The figure shows three views and two pictorial views of one solid part (mm, origin at its lowest corner). Answer the questions. A direction names the side the tool comes from. Round coordinates to 2 decimals unless told otherwise and drop trailing zeros. Order: outer loops, then holes, each group sorted by start corner. A loop starts at its lowest first (then second) coordinate and runs counter-clockwise, first axis right, second up. Notation, with made-up numbers: M 27.5,-12.75 L 53.5,-12.75 A24 cw 53.5,13.25 Z; hole C 38.25,0.5 d8. An arc over 180 degrees is marked long. Answer as CSV lines item,"result".
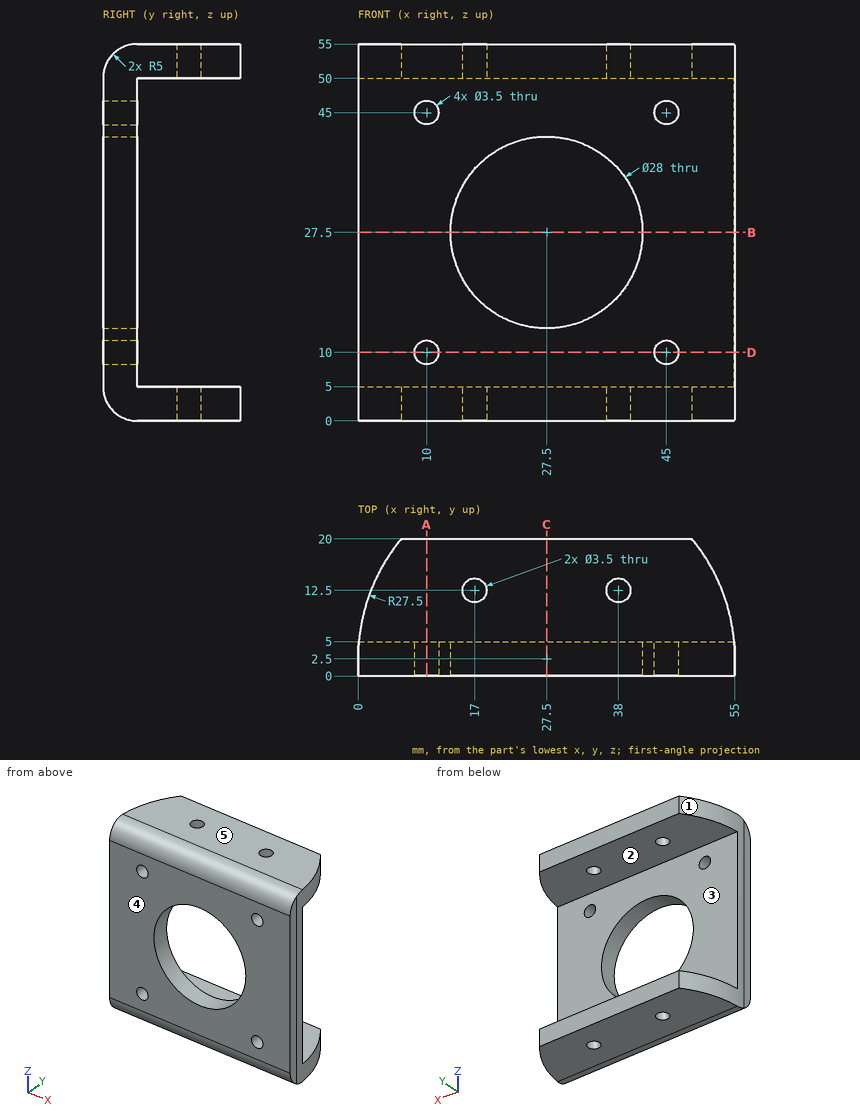
Item 1: A cutting plane is placed at D-D, the plane z = 10. Determine the outline of the cut face in (x, y), and give its area (3 significant figures).
Ans:
outline,"M 0,0 L 8.25,0 L 8.25,5 L 0.11,5 A27.5 ccw 0,2.5 Z; M 11.75,0 L 43.25,0 L 43.25,5 L 11.75,5 Z; M 46.75,0 L 55,0 L 55,2.5 A27.5 ccw 54.89,5 L 46.75,5 Z"
area,"240 mm2"
Item 2: A cutting plane is placed at A-A, the plane x = 10. Determine the outline of the cut face in (y, z), and give its area (3 significant figures).
Ans:
outline,"M 0,5 A5 ccw 5,0 L 20,0 L 20,5 L 5,5 L 5,8.25 L 0,8.25 Z; M 0,11.75 L 5,11.75 L 5,43.25 L 0,43.25 Z; M 0,46.75 L 5,46.75 L 5,50 L 20,50 L 20,55 L 5,55 A5 ccw 0,50 Z"
area,"379 mm2"
Item 3: A cutting plane is placed at C-C, the plane x = 27.5. Determine the outline of the cut face in (y, z).
Ans:
outline,"M 0,5 A5 ccw 5,0 L 20,0 L 20,5 L 5,5 L 5,13.5 L 0,13.5 Z; M 0,41.5 L 5,41.5 L 5,50 L 20,50 L 20,55 L 5,55 A5 ccw 0,50 Z"
Item 4: Flat-ended cylindrical pins translate along their axes: pin 1 (22.5 mm diameter, centred on x = 21.5, z = 32, fed in from +Y); pin 2 (3 mm diameter, centred on x = 45, z = 45, fed in from +Y); pin 3 (8 mm diameter, centred on y = 13.5, z = 7, fed in from +X); pin 4 (3 mm diameter, centred on y = 5.5, z = 15, fed in from +X). Find the tip coordinate at first contact, or state that the pin passes through.
Ans:
pin 1,"y = 5"
pin 2,"through"
pin 3,"x = 53.95"
pin 4,"x = 54.96"
Item 5: Find the intervals of material crossed by probe 1 along Z at (x, y) = (22.5, 19); probe 2 along X at (y, z) = (1.25, 11.5); probe 3 along Z at (x, y) = (10, 1.1), in increasing order. Write a range as [from, to].
Ans:
probe 1,"[0, 5], [50, 55]"
probe 2,"[0, 9.1], [10.9, 44.1], [45.9, 55]"
probe 3,"[1.87, 8.25], [11.75, 43.25], [46.75, 53.13]"
Item 6: Determine the mould class of the marked faces 3, 4 and 5 for opening direction Z: +Z half, -Z half, draft (parallel to the pull), parting line (faces both ways), or undercut.
Ans:
face 3,"undercut"
face 4,"draft"
face 5,"+Z half"
Item 7: A tool of negligible diameter and unlimited length cuts with its end or side. For the marked faces 1 and 2, from which of +Z, -Z, +X, -X, +Y, -Y can it reach the whole face along a straight path? Write none if from no direction.
Ans:
face 1,"+Z, -Z, -X, +Y"
face 2,"+X, -X, +Y"
Item 8: A cutting plane is placed at B-B, the plane z = 27.5. Determine the outline of the cut face in (x, y), and give its area (3 significant figures).
Ans:
outline,"M 0,0 L 13.5,0 L 13.5,5 L 0.11,5 A27.5 ccw 0,2.5 Z; M 41.5,0 L 55,0 L 55,2.5 A27.5 ccw 54.89,5 L 41.5,5 Z"
area,"135 mm2"
